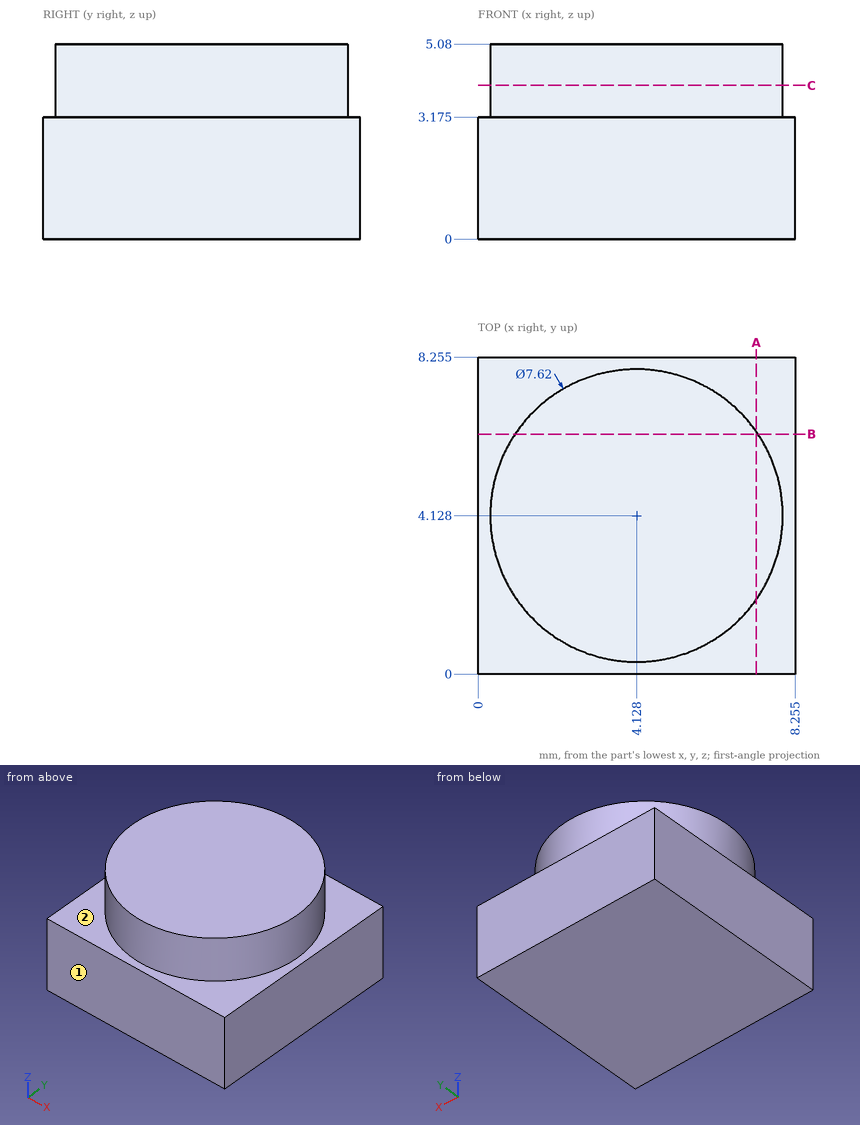
Can you work these out from the drawing? Everything is in mm from the part's minimum corner. A direction names the side the tool comes from. Give positions to 0.01 mm unless a question says otherwise; leave off trailing zeros. Order: outer loops, then holes, each group sorted by start corner. A loop starts at its lowest first (then second) coordinate and runs counter-clockwise, first axis right, second up. Notation, with made-up numbers: M 19.5,75.25 L 44.5,75.25 A22 ccw 44.5,94.25 Z; hole C 21.25,30.5 d8. An arc over 180 degrees is marked long. Write item = value, one per line. Start each with the question number.
Q1. I need wall thicknesses on probe 1 along Z at (x, y) = (0.5, 7) (1 decimal); probe 2 along Y at (x, z) = (4.25, 3.45) (1 decimal); probe 3 along X at (y, z) = (5.75, 3.7) (1 decimal). Which ranges of each line are inside material? Lowest first, please. Write a range as [from, to].
Q2. Suppose I cut it at C-C (z = 4). Write out the boundary of the cut face in (x, y).
Q3. For the marked faces 1 and 2, which set-ups out of +Z, -Z, +X, -X, +Y, -Y let a thin tool reach every point of the face, with its end or its side?
Q4. Suppose I cut it at A-A (x = 7.25). Write out the boundary of the cut face in (y, z) (1 decimal).
Q5. Suppose I cut it at B-B (y = 6.25). Write out the boundary of the cut face in (x, z) (1 decimal).
Check result:
q1.probe_1 = [0, 3.2]
q1.probe_2 = [0.3, 7.9]
q1.probe_3 = [0.7, 7.6]
q2.outline = C 4.13,4.13 d7.62
q3.face_1 = +Z, -Z, +X, -X, -Y
q3.face_2 = +Z
q4.outline = M 0,0 L 8.3,0 L 8.3,3.2 L 6.3,3.2 L 6.3,5.1 L 1.9,5.1 L 1.9,3.2 L 0,3.2 Z
q5.outline = M 0,0 L 8.3,0 L 8.3,3.2 L 7.3,3.2 L 7.3,5.1 L 1,5.1 L 1,3.2 L 0,3.2 Z
